from build123d import *

# Parameters (mm, degrees)
SKETCH1_R           = 0.5
SKETCH1_R_2         = 0.429709329
BOSS_EXTRUDE1_DEPTH = 5


with BuildPart() as part:
    # Sketch1 → Boss-Extrude1 (new body)
    with BuildSketch(Plane.XY):
        with BuildLine():
            Line((85, 0), (85, -6.75))
            Line((85, -6.75), (112.500186095, -6.75))
            Line((112.500186095, -6.75), (112.500186095, -23.25))
            Line((112.500186095, -23.25), (77.499813905, -23.25))
            Line((77.499813905, -23.25), (75, -23.25))
            Line((75, -23.25), (75, 0))
            ThreePointArc((75, 0), (37.5, 37.5), (0, 0))
            ThreePointArc((0, 0), (-5, -5), (-10, 0))
            ThreePointArc((-10, 0), (37.5, 47.5), (85, 0))
        make_face()
        with Locations((95, -8.25)):
            Circle(SKETCH1_R, mode=Mode.SUBTRACT)
        with Locations((95, -10.75)):
            Circle(SKETCH1_R_2, mode=Mode.SUBTRACT)
        with Locations((95, -21.73)):
            Circle(SKETCH1_R, mode=Mode.SUBTRACT)
        with Locations((95, -19.23)):
            Circle(SKETCH1_R, mode=Mode.SUBTRACT)
        with Locations((111.000186095, -15)):
            Circle(SKETCH1_R, mode=Mode.SUBTRACT)
        with Locations((108.500186095, -15)):
            Circle(SKETCH1_R, mode=Mode.SUBTRACT)
        with Locations((81.500186095, -15)):
            Circle(SKETCH1_R, mode=Mode.SUBTRACT)
        with Locations((79.000186095, -15)):
            Circle(SKETCH1_R, mode=Mode.SUBTRACT)
    extrude(amount=BOSS_EXTRUDE1_DEPTH)


solid = part.part
Verification items for the finished model (mm, model axes). A direction names the side the tool comes from. Give positions to 0.01 mm unless a question says otherwise; leave off trailing zeros. Write each loop counter-clockwise with the first axis right and the second up, starting at its lowest first coordinate (ties: lowest second). Pieces come first, ordered by that corner, then holes. Notation, with made-up numbers: M 16.25,26 L 34.25,26 A20 ccw 34.25,52 Z; hole C -25,-19 d6. An arc over 180 degrees is marked long. Use CSV: the item, a comma, the result in double quotes.
1) Go/stop test with flat-tipped pins: pin 1 Ø3 at (y, z) = (-1, 4.5) entering from +X; pin 2 Ø1 at (x, z) = (95.5, 3) entering from +Y. Record where each tip stops, or that it passes through.
Final values:
pin 1,"x = 85"
pin 2,"y = -6.75"
2) Cross-section at D-D (y = 6.5). Enter the section's corners in (x, z).
Final values:
outline,"M -9.55,0 L 0.57,0 L 0.57,5 L -9.55,5 Z; M 74.43,0 L 84.55,0 L 84.55,5 L 74.43,5 Z"
3) Cross-section at C-C (x = 37.5). Enter the section's corners in (y, z), plus the area to 3 significant figures.
Final values:
outline,"M 37.5,0 L 47.5,0 L 47.5,5 L 37.5,5 Z"
area,"50.0 mm²"
4) Material ranges on line 1 along Y through (x, z) = (95, 3.15); line 2 along X through (y, z) = (-16.5, 1.6); line 3 along X through (y, z) = (26, 0.55), recorded low to high.
Final values:
line 1,"-23.25 to -22.23, -21.23 to -19.73, -18.73 to -11.18, -10.32 to -8.75, -7.75 to -6.75"
line 2,"75 to 112.5"
line 3,"-2.25 to 10.48, 64.52 to 77.25"
5) Cross-section at A-A (y = 27.5). Enter the section's corners in (x, z), plus the area to 3 significant figures.
Final values:
outline,"M -1.23,0 L 12,0 L 12,5 L -1.23,5 Z; M 63,0 L 76.23,0 L 76.23,5 L 63,5 Z"
area,"132 mm²"
6) Access from +Z, -Z, +X, -X, +Y, -Y to the whole of each face (thin tool, end or side, straight path). Record for faces 1 (the face through (85, -3, 2)), 2 (the face through (75, -12, 2)), 3 (the face through (70, 20, 0)).
Final values:
face 1,"+Z, -Z, +X, +Y"
face 2,"+Z, -Z, -Y"
face 3,"-Z, +X, -X, +Y, -Y"
7) Cross-section at B-B (z = 1). State how many separate pieces and enclosed holes the cut face has, plus the area to 3 significant figures.
Final values:
separate pieces,"1"
enclosed holes,"8"
area,"2,050 mm²"
